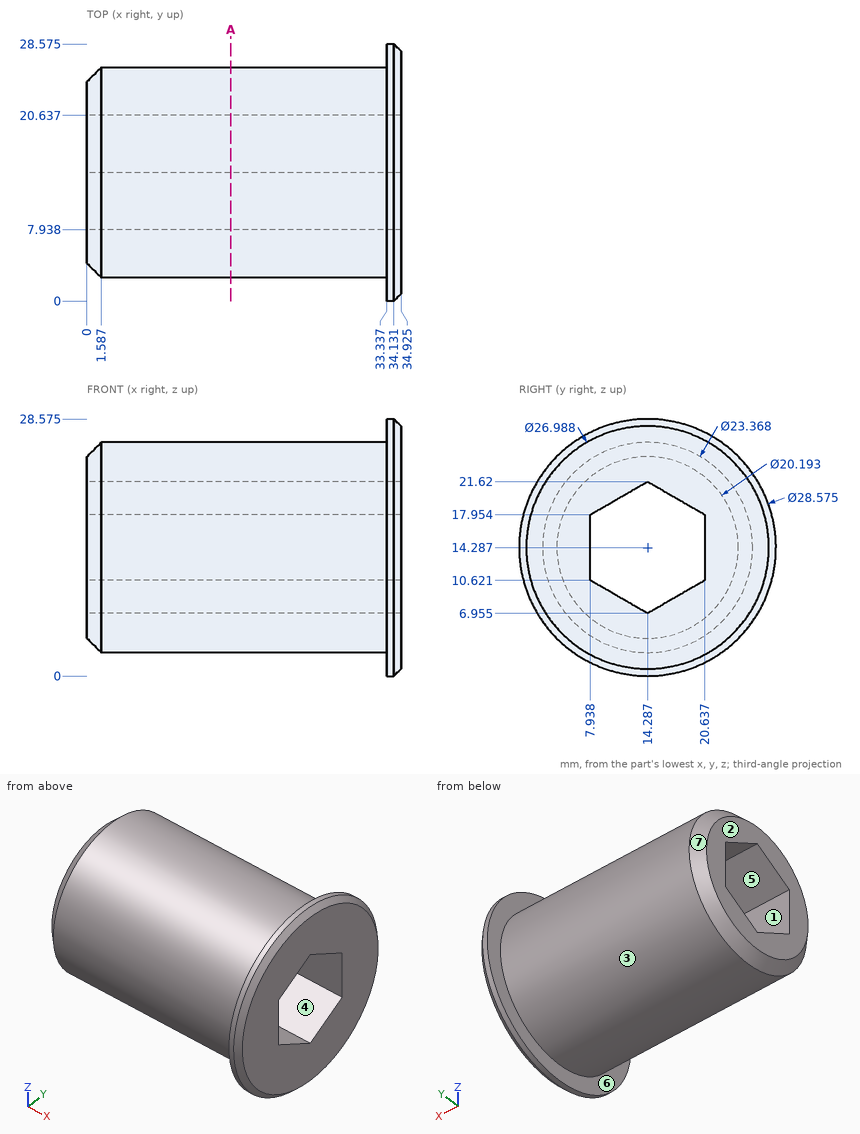
Could you check a few things on this drawing? It's one solid part, dimensions in mm from its lowest x, y, z. A direction names the side the tool comes from. Coordinates: 2 decimals unless noted, no trailing zeros. Write each loop counter-clockwise with the first axis right and the second up, starting at its lowest first coordinate (ties: lowest second). Pieces come first, ordered by that corner, then holes. Notation, with made-up numbers: (38, -0.75) - (65, -0.75) arc R18 ccw to (65, 20.25) - close; hole circle Ø6 at (-29.5, 56.5). An arc over 180 degrees is marked (long way). Use one line per item in the form item = value.
1) Thinking about a two-plate mould opening in Y: for the marked faces 4, 5, 6 and 7, which applies, released by +Y, released by -Y, zero draft, split by the parting line, or undercut?
Solved:
face_4 = undercut
face_5 = undercut
face_6 = zero draft
face_7 = split by the parting line
2) I need wall thicknesses on line 1 (Y direction, x = 30.5, z = 14.5) (1 decimal); line 2 (Z direction, x = 19, y = 9.5) (1 decimal); line 3 (Y direction, x = 19, z = 12) (1 decimal). Which ranges of each line are inside material? Lowest first, please.
Solved:
line_1 = 2.6 to 7.9, 20.6 to 26
line_2 = 3.6 to 9.7, 18.9 to 24.9
line_3 = 2.8 to 7.9, 20.6 to 25.7
3) On a 3-axis mill with a long thin cutter (end or side, diameter ignored), from which of +Z, -Z, +X, -X, +Y, -Y can I reach the whole of each face in a straight line? I mean the marked faces 1, 2 and 3. Say none if no direction works.
Solved:
face_1 = +X, -X
face_2 = +Z, -Z, -X, +Y, -Y
face_3 = -X
4) Suppose I cut it at A-A, the plane x = 16. Write out the boundary of the cut face in (y, z) (1 decimal), plus the area to 3 significant figures.
Solved:
outline = circle Ø23.4 at (14.3, 14.3); hole (7.9, 10.6) - (14.3, 7) - (20.6, 10.6) - (20.6, 18) - (14.3, 21.6) - (7.9, 18) - close
area = 289 mm2
5) I'm going to push flat-ended pins straight in: P1, Ø3, axis at x = 11, z = 12, coming from the +Y side (1 decimal); P2, Ø1, axis at x = 5.5, z = 25, coming from the +Y side (1 decimal); P3, Ø8, axis at x = 20.5, y = 21, coming from the -Z side; P4, Ø1.5, axis at y = 22, z = 9.5, coming from the -X side. Where does each tip first touch, or does it pass through?
Solved:
P1 = 25.9
P2 = 20
P3 = 2.92
P4 = 0
